Verification items for the finished model (mm, model axes). Face numbers are marked on the shaded views. A direction names the side the tool comes from. Coordinates: 2 decimals unless noted, no trailing zeros. Order: outer loops, then holes, each group sorted by start corner. A loop starts at its lowest first (then second) coordinate and runs counter-clockwise, first axis right, second up.
Q1. Cross-section at A-A, the plane x = 0. Record the boundary of the cut face in (y, z).
Q2. Thickness scan on line 1 (X direction, y = -1.25, z = 8); line 2 (X direction, y = 0, z = -9.5). Record the ranges inside material, lowest first.
Q3. Set-up check for the marked faces 1 and 2: record each of +Z, -Z, +X, -X, +Y, -Y from which the full face is reachable in a straight line by a thin tool's end or side.
Q4. Cross-section at B-B, the plane z = -9. Record the boundary of the cut face in (x, y), and give its area (3 significant figures).
Q5. Depth check by flat-ended pin: P1, Ø0.7, axis at x = 3, z = 12.5, coming from the +Y side; P2, Ø1, axis at y = -0.5, z = 5, coming from the -X side; P3, Ø3, axis at y = 0, z = 10, coming from the +X side. Enter the tip coordinate at first touch or a pass-through.
Autodesk Inventor part; units mm, degrees
ref_plane "Work Plane6" through (0, 0, 8) normal (0, 0, 1) x (1, 0, 0)
ref_plane "Work Plane7" through (0, -4.8919, 8) normal (1, 0, 0) x (0, 1, 0)
ref_plane "YZ Plane" through (0, 0, 0) normal (1, 0, 0) x (0, 1, 0)
sketch "Sketch1" plane through (0, 0, 0) normal (0, 0, 1) x (1, 0, 0)
  circle A0 centre (0, 0) radius 12
  circle A1 centre (0, 0) radius 1.5
  dimension "d0" = 24
  dimension "d2" = 3
extrude "Extrusion1" add sketch "Sketch1" along normal blind 3
sketch "Sketch2" plane through (0, 0, 3) normal (0, 0, 1) x (1, 0, 0)
  circle A0 centre (0, 0) radius 1.5
  circle A1 centre (0, 0) radius 12
  circle A2 centre (0, 0) radius 5
  dimension "d5" = 10
extrude "Extrusion2" add sketch "Sketch2" along normal blind 10 contours A2
sketch "Sketch14" plane through (0, 0, 0) normal (0, 0, -1) x (-1, 0, 0)
  circle A0 centre (0, 0) radius 1.5
  circle A1 centre (0, 0) radius 12
extrude "Extrusion11" add sketch "Sketch14" along normal blind 20
ref_plane "Work Plane6" through (0, 0, 8) normal (0, 0, 1) x (1, 0, 0)
sketch "Sketch15" plane through (0, 0, 8) normal (0, 0, 1) x (1, 0, 0)
  line L0 (0, -4.8919) -> (0, 6.5751)
  point P0 (0, 0)
ref_plane "Work Plane7" through (0, -4.8919, 8) normal (1, 0, 0) x (0, 1, 0)
fillet "Fillet3" radius 5 1 edges at (-5, 0, 3)
fillet "Fillet4" radius 5 1 edges at (-12, 0, 3)
sketch "Sketch17" plane through (0, 0, 13) normal (0, 0, 1) x (1, 0, 0)
  circle A0 centre (0, 0) radius 1.5
  circle A1 centre (0, 0) radius 5
  line L0 (0, -5) -> (0, 5)
ref_plane "Work Plane8" through (0, -5, 13) normal (1, 0, 0) x (0, 1, 0)
sketch "Sketch18" plane through (0, -5, 13) normal (1, 0, 0) x (0, 1, 0)
  circle A0 centre (5, -3) radius 1.3323
  line L0 (10, 0) -> (0, 0)
  point P0 (5, -13)
  dimension "d88" = 3
extrude "Extrusion13" cut sketch "Sketch18" along normal blind 10
sketch "Sketch19" plane through (0, 0, 13) normal (0, 0, 1) x (1, 0, 0)
  circle A0 centre (0, 0) radius 1.5
  line L0 (2, -2.75) -> (3.6, -2.75)
  line L1 (3.6, -2.75) -> (3.6, 2.75)
  line L2 (3.6, 2.75) -> (2, 2.75)
  line L3 (2, 2.75) -> (2, -2.75)
  dimension "d91" = 5.5
  dimension "d93" = 2.75
  dimension "d94" = 1.6
  dimension "d95" = 2
ref_plane "Work Plane9" through (2, 2.75, 13) normal (1, 0, 0) x (0, -1, 0)
sketch "Sketch20" plane through (2, 2.75, 13) normal (1, 0, 0) x (0, -1, 0)
  line L0 (2.75, 6.1546) -> (5.5, 4.5669)
  line L1 (5.5, 4.5669) -> (5.5, 1.3914)
  line L2 (5.5, 1.3914) -> (2.75, -0.1963)
  line L3 (2.75, -0.1963) -> (0, 1.3914)
  line L4 (0, 1.3914) -> (0, 4.5669)
  line L5 (0, 4.5669) -> (2.75, 6.1546)
  point P0 (2.75, 13)
  point P1 (2.75, 2.9792)
  dimension "d97" = 5.5
extrude "Extrusion14" cut sketch "Sketch20" along normal blind 1.6
sketch "Sketch21" plane through (0, 0, 13) normal (0, 0, 1) x (1, 0, 0)
  line L0 (2, 0.34) -> (3.6, 0.34)
  line L1 (3.6, 0.34) -> (3.6, -0.34)
  line L2 (3.6, -0.34) -> (2, -0.34)
  line L3 (2, -0.34) -> (2, 0.34)
  circle A0 centre (0, 0) radius 1.5
  circle A1 centre (0, 0) radius 5
  line L4 (2, -2.7571) -> (3.6, -2.7571)
  line L5 (3.6, -2.7571) -> (3.6, 2.7571)
  line L6 (3.6, 2.7571) -> (2, 2.7571)
  line L7 (2, 2.7571) -> (2, -2.7571)
extrude "Extrusion15" cut sketch "Sketch19" against normal blind 3 contours L3 L2 L1 L0
properties part number "support shaft end"
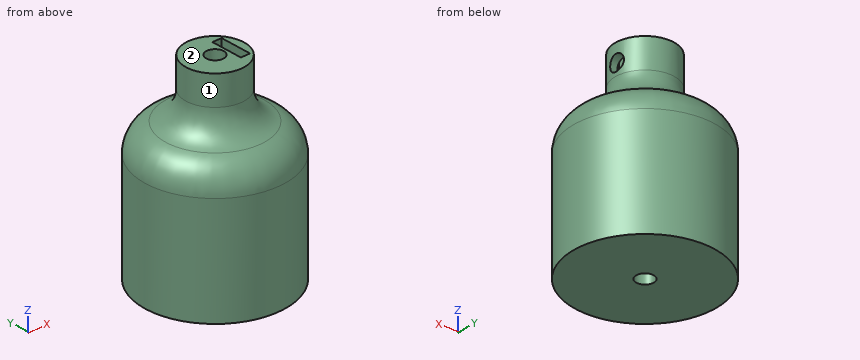
Check values:
1. outline: (-12, -20) - (-1.5, -20) - (-1.5, 13) - (-5, 13) - (-5, 8) arc R5 cw to (-8.5, 3.23) arc R5 ccw to (-12, -1.54) - close; (1.5, -20) - (12, -20) - (12, -1.54) arc R5 ccw to (8.5, 3.23) arc R5 cw to (5, 8) - (5, 13) - (1.5, 13) - close
2. line 1: x = -4.84 to -0.83, 0.83 to 2, 3.6 to 4.84
2. line 2: x = -12 to -1.5, 1.5 to 12
3. face 1: +Z
3. face 2: +Z, +X, -X, +Y, -Y
4. outline: circle Ø24 at (0, 0); hole circle Ø3 at (0, 0)
4. area: 445 mm2
5. P1: stops at y = 4.24
5. P2: stops at x = -6.41
5. P3: stops at x = 5
